Could you check a few things on this drawing? It's one solid part, dimensions in mm from its lowest x, y, z. A direction names the side the tool comes from. Give positions to 0.01 mm unless a question says otherwise; leave off trailing zeros. Order: outer loops, then holes, each group sorted by start corner. A loop starts at its lowest first (then second) coordinate and runs counter-clockwise, first axis right, second up. Notation, with made-up numbers: (-17, -38.75) -> (37, -38.75) arc R24 cw to (37, -23.75) -> close; hole circle Ø7 at (77, -4). An arc over 180 degrees is marked (long way). Answer as CSV lines item,"result".
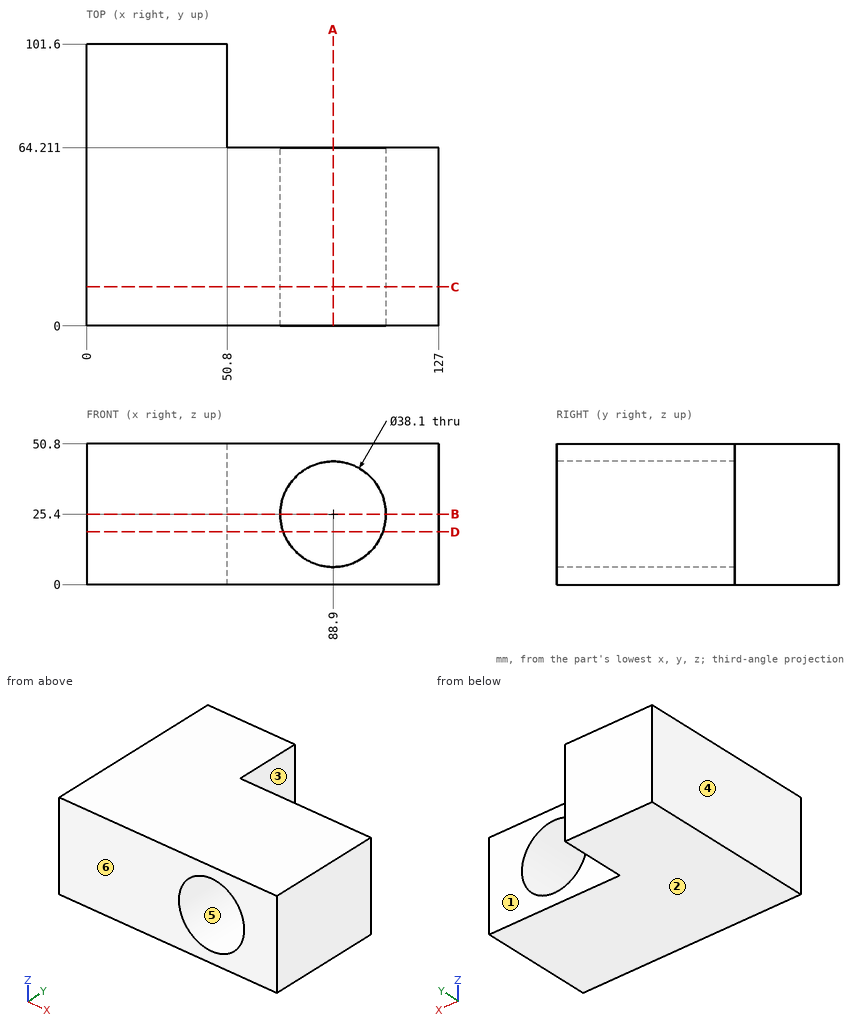
Item 1: For pin 1 (23 mm diameter, centred on x = 88.9, z = 25.4, fed in from -Y); pin 2 (3 mm diameter, centred on y = 85, z = 29.5, fed in from +X); pin 3 (10 mm diameter, centred on y = 88, z = 27, fed in from -X), each with a flat end and sliding along its axis, tell me the tip position at first contact or that it passes through.
Numbers:
pin 1,"passes through"
pin 2,"stops at x = 50.8"
pin 3,"stops at x = 0"
Item 2: Imagine slicing it at B-B, the plane z = 25.4. Please give me the cut outline in (x, y).
Numbers:
outline,"(0, 0) -> (69.85, 0) -> (69.85, 64.21) -> (50.8, 64.21) -> (50.8, 101.6) -> (0, 101.6) -> close; (107.95, 0) -> (127, 0) -> (127, 64.21) -> (107.95, 64.21) -> close"
Item 3: Imagine slicing it at A-A, the plane x = 88.9. Please give me the cut outline in (y, z).
Numbers:
outline,"(0, 0) -> (64.21, 0) -> (64.21, 6.35) -> (0, 6.35) -> close; (0, 44.45) -> (64.21, 44.45) -> (64.21, 50.8) -> (0, 50.8) -> close"
Item 4: We'd pull the mould along X, two halves only. Please class the marked faces 3, 4, 5 and 6: released by +X, released by -X, zero draft, split by the parting line, or undercut.
Numbers:
face 3,"released by +X"
face 4,"released by -X"
face 5,"undercut"
face 6,"zero draft"
Item 5: For the marked faces 1 and 2, which set-ups out of +Z, -Z, +X, -X, +Y, -Y let a thin tool reach every point of the face, with its end or its side?
Numbers:
face 1,"+Z, -Z, +X, +Y"
face 2,"-Z, +X, -X, +Y, -Y"
Item 6: Imagine slicing it at D-D, the plane z = 19. Please give me the cut outline in (x, y).
Numbers:
outline,"(0, 0) -> (70.96, 0) -> (70.96, 64.21) -> (50.8, 64.21) -> (50.8, 101.6) -> (0, 101.6) -> close; (106.84, 0) -> (127, 0) -> (127, 64.21) -> (106.84, 64.21) -> close"
Item 7: Imagine slicing it at C-C, the plane y = 14. Please give me the cut outline in (x, z), then the cut area to 3 significant figures.
Numbers:
outline,"(0, 0) -> (127, 0) -> (127, 50.8) -> (0, 50.8) -> close; hole circle Ø38.1 at (88.9, 25.4)"
area,"5,310 mm²"
Item 8: Please list where these lines run through material, in increasing order: line 1 along X through (y, z) = (37, 25.4); line 2 along Z through (x, y) = (88.9, 40); line 3 along X through (y, z) = (90, 35.5).
Numbers:
line 1,"x = 0 to 69.85, 107.95 to 127"
line 2,"z = 0 to 6.35, 44.45 to 50.8"
line 3,"x = 0 to 50.8"
